```python
from build123d import *

# Parameters (mm, degrees)
BOSS_EXTRUDE1_DEPTH = 18
CHAMFER1_SIZE       = 2


with BuildPart() as part:
    # Sketch1 → Boss-Extrude1 (new, symmetric)
    with BuildSketch(Plane.XY):
        Polygon((28, 55), (-28, 55), (-28, -55), (28, -55), (28, -37.1), (-9.2, -37.1), (-9.2, -18), (28, -18), (28, 18), (-9.2, 18), (-9.2, 37.1), (28, 37.1), align=None)
    extrude(amount=BOSS_EXTRUDE1_DEPTH, both=True)

    # Chamfer1
    chamfer1_edges = [part.edges().sort_by_distance(p)[0] for p in [
        (-28, 0, 18),
        (0, -55, -18),
        (-28, 0, -18),
        (0, 55, -18),
        (0, -55, 18),
        (-28, -55, 0),
        (-28, 55, 0),
        (0, 55, 18),
    ]]
    chamfer(chamfer1_edges, length=CHAMFER1_SIZE)


solid = part.part
```
Work out the finished part from the listing and answer in its coordinate system (mm). A direction names the side the tool comes from. Give positions to 0.01 mm unless a question says otherwise; leave off trailing zeros. Write each loop counter-clockwise with the first axis right and the second up, starting at its lowest first coordinate (ties: lowest second). Pieces come first, ordered by that corner, then holes.
(1) The part is cut by section B-B on z = -6. Write down the section's boundary in (x, y).
Final values:
outline: (-28, -53) - (-26, -55) - (28, -55) - (28, -37.1) - (-9.2, -37.1) - (-9.2, -18) - (28, -18) - (28, 18) - (-9.2, 18) - (-9.2, 37.1) - (28, 37.1) - (28, 55) - (-26, 55) - (-28, 53) - close
(2) Which of the six approach directions +Z, -Z, +X, -X, +Y, -Y give full straight-line access (tool end or side, diameter ignored) to faces 4 (the flat face through (28, 46, 0)), 5 (the flat face through (-9.2, -28, 0))?
Final values:
face 4: +Z, -Z, +X, +Y, -Y
face 5: +Z, -Z, +X
(3) Straight lines are drawn through the part: line 1 (Y direction, x = 4.5, z = -1.5); line 2 (X direction, y = -20.5, z = 12). For each, find the intervals that lie inside material, in ascending order.
Final values:
line 1: y = -55 to -37.1, -18 to 18, 37.1 to 55
line 2: x = -28 to -9.2
(4) Flat-ended cylindrical pins translate along their axes: pin 1 Ø15.5 at (y, z) = (26.5, 8) entering from +X; pin 2 Ø21 at (y, z) = (-24, 4) entering from +X. Find the tip coordinate at first contact, or state that the pin passes through.
Final values:
pin 1: stops at x = -9.2
pin 2: stops at x = 28
(5) The part is cut by section C-C on y = 24. Write down the section's boundary in (x, z).
Final values:
outline: (-28, -16) - (-26, -18) - (-9.2, -18) - (-9.2, 18) - (-26, 18) - (-28, 16) - close
(6) The mould has two halves that part along Y. Classify faces 1 (the flat face through (9, 37.1, 0)), 2 (the flat face through (-28, 1, 0)), 3 (the flat face through (-27, 54, 0)): pulls with the +Y half, pulls with the -Y half, needs draft (parallel to the pull), parting line crosses it, or undercut.
Final values:
face 1: undercut
face 2: needs draft
face 3: pulls with the +Y half
(7) The part is cut by section A-A on x = 1. Write down the section's boundary in (y, z), plus the area to 3 significant figures.
Final values:
outline: (-55, -16) - (-53, -18) - (-37.1, -18) - (-37.1, 18) - (-53, 18) - (-55, 16) - close; (-18, -18) - (18, -18) - (18, 18) - (-18, 18) - close; (37.1, -18) - (53, -18) - (55, -16) - (55, 16) - (53, 18) - (37.1, 18) - close
area: 2,580 mm2
